Design review of the part shown in the three views and the two pictorial views. Dimensions are in mm from the part's minimum x, y and z. Round coordinates to 2 decimals unless told otherwise and drop trailing zeros. Order: outer loops, then holes, each group sorted by start corner. A loop starts at its lowest first (then second) coordinate and runs counter-clockwise, first axis right, second up. Notation, with made-up numbers: M 88.25,-22.5 L 146.25,-22.5 A15 cw 146.25,-4.5 Z; hole C 1,76.25 d10. An arc over 180 degrees is marked long. Write each question's results on one line, items separated by ' | '. Start each with the question number.
Item 1: Take a section at A-A, the plane y = 152.4. Write out the cut boundary in (x, z).
Item 2: The part is to be moulded in two halves that separate along Z. For the marked faces 1, 2 and 3, say which applies: +Z half, -Z half, draft (parallel to the pull), parting line (faces both ways), or undercut.
Item 3: Clearance check with flat-ended pins moving along their axes: pin 1 (12 mm diameter, centred on x = 792, z = 206, fed in from -Y); pin 2 (5 mm diameter, centred on y = 245, z = 273, fed in from -X); pin 3 (1 mm diameter, centred on x = 386, y = 161.5, fed in from -Z). State where each tip first meets the part, or that it passes through.
Item 4: Take a section at B-B, the plane x = 278. Write out the cut boundary in (y, z), plus the area to 3 significant figures.
Item 5: Take a section at D-D, the plane z = 252. Write out the cut boundary in (x, y).
Item 6: Wall thickness on line 1 (X direction, y = 213, z = 152); line 2 (Z direction, x = 937, y = 152); line 3 (Y direction, x = 616, z = 87.5): over which ranges is each line inside the solid? List them lowest first. Write a range as [from, to].
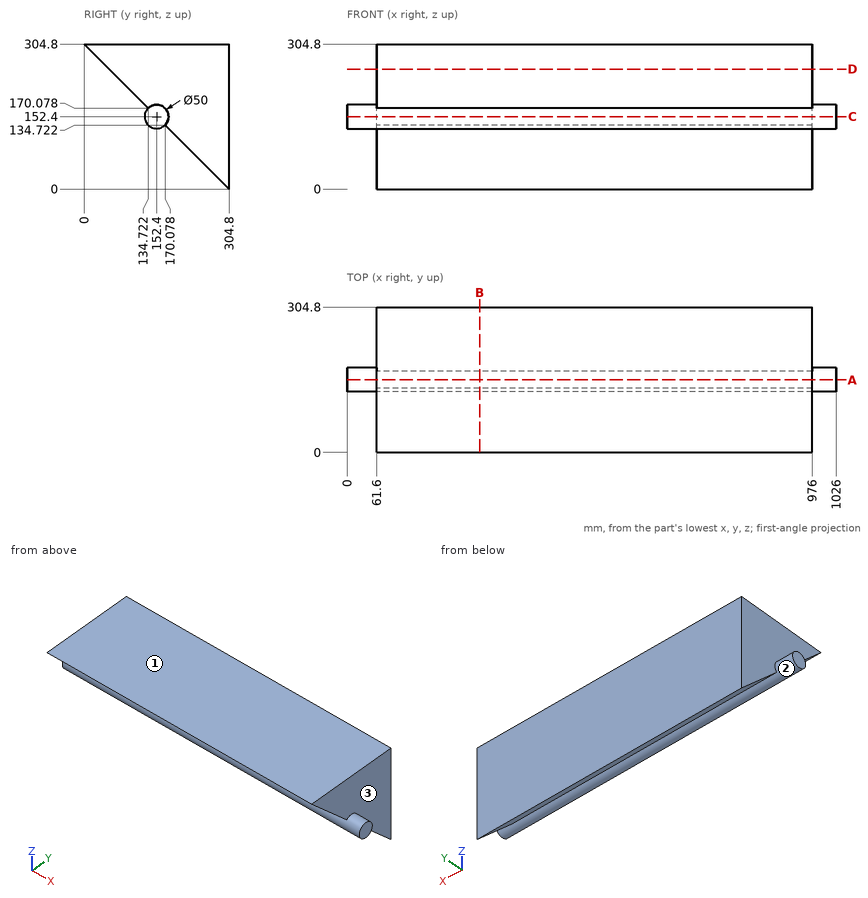
Results list:
1) outline: M 0,127.4 L 1026,127.4 L 1026,177.4 L 976,177.4 L 976,304.8 L 61.6,304.8 L 61.6,177.4 L 0,177.4 Z
2) face 1: +Z half | face 2: undercut | face 3: draft
3) pin 1: y = 92.8 | pin 2: x = 61.6 | pin 3: z = 128.93
4) outline: M 0,304.8 L 134.72,170.08 A25 ccw 170.08,134.72 L 304.8,0 L 304.8,304.8 Z | area: 47,400 mm²
5) outline: M 61.6,52.8 L 976,52.8 L 976,304.8 L 61.6,304.8 Z
6) line 1: [61.6, 976] | line 2: [127.4, 304.8] | line 3: [217.3, 304.8]
